Geometry: see drawing. Coordinates: mm, zero at the bounding-box minimum. A direction names the side the tool comes from. Coordinates: 2 decimals unless noted, no trailing zeros. Write each loop counter-clockwise with the first axis right and the second up, starting at its lowest first coordinate (ties: lowest second). Pieces come first, ordered by that corner, then holes. Notation, with made-up numbers: M -30.75,-38 L -4.75,-38 A20 ccw -4.75,-33 Z; hole C -23,-12 d3. An arc over 180 degrees is marked long. Answer as CSV lines item,"result". Start each with the question number.
1. Line query: probe 1 along Y at (x, z) = (22, 16.25) (1 decimal); probe 2 along Y at (x, z) = (8.75, 6.5) (1 decimal); probe 3 along X at (y, z) = (7.5, 13.75) (1 decimal). Output: solid intervals per line, ascending. Write a range as [from, to].
2. Contact query for flat-ended pins moving along their axis: pin 1 Ø1 at (y, z) = (14, 15) entering from +X; pin 2 Ø0.8 at (x, z) = (28, 6.5) entering from +Y (3 decimals); pin 3 Ø1.3 at (y, z) = (12, 10.5) entering from -X; pin 4 Ø1.6 at (x, y) = (2.125, 5.7) entering from +Z. Output: stop coordinate, or through.
3. Section D-D on y = 5.7. Return the cut outline in (x, z) (1 decimal), plus the area to 3 significant figures.
4. Section C-C on x = 24. Return the cut outline in (y, z) (1 decimal).
5. Section A-A on z = 2.25. Count the separate pieces of the cut face and the enclosed holes in it, plus the area to 3 significant figures.
6. Section B-B on y = 14.75. Return the cut outline in (x, z) (1 decimal), plus the area to 3 significant figures.
7. Mould query, pull axis Z, two halves, no side actions, for the marked faces 4, 5 and 6. Classes: pulls with the +Z half, pulls with the -Z half, needs draft (parallel to the pull), parting line crosses it, or undercut.
8. Reachability of the marked faces 1, 2 and 3 from +Z, -Z, +X, -X, +Y, -Y: full face, straight path, thin tool, end or side. Return the list, or none.
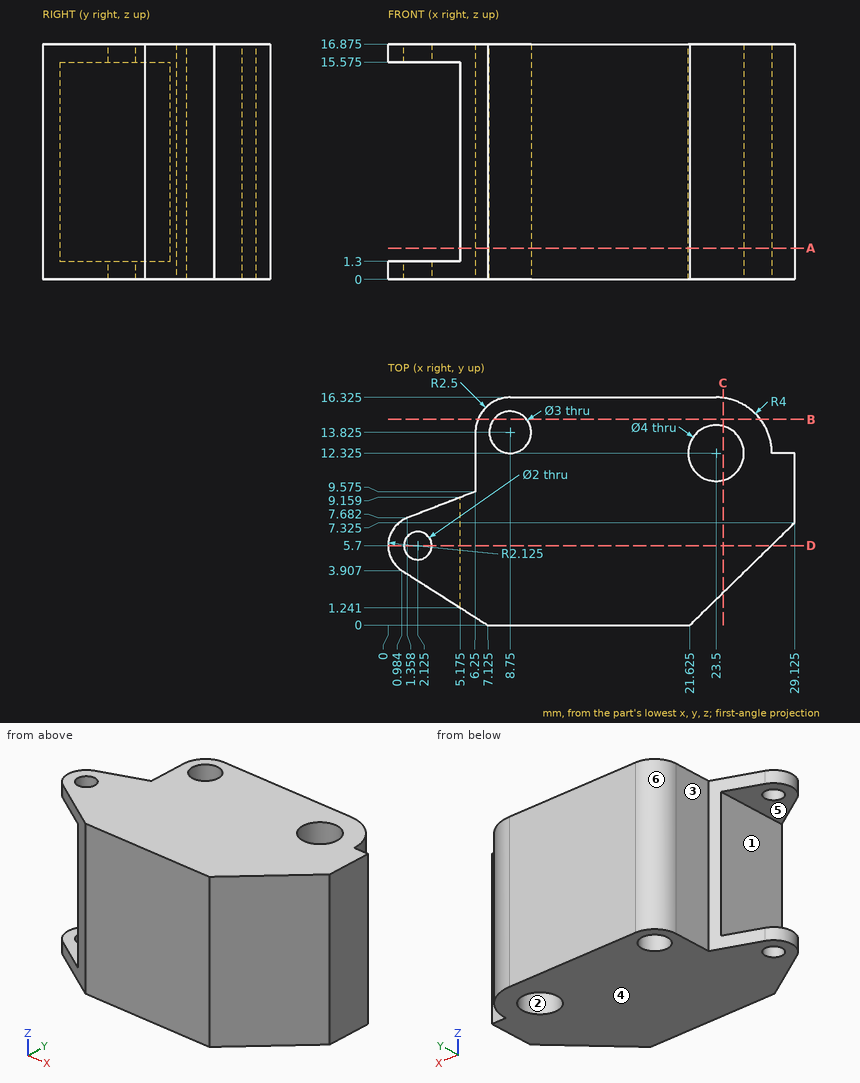
Values:
1,probe 1,"[0.4, 11], [13.6, 16.3]"
1,probe 2,"[0, 12.3], [15.3, 16.3]"
1,probe 3,"[5.2, 29.1]"
2,pin 1,"x = 27.32"
2,pin 2,"y = 12.325"
2,pin 3,"x = 6.25"
2,pin 4,"through"
3,outline,"M 0,0 L 1.1,0 L 1.1,1.3 L 0,1.3 Z; M 0,15.6 L 1.1,15.6 L 1.1,16.9 L 0,16.9 Z; M 3.1,0 L 27.5,0 L 27.5,16.9 L 3.1,16.9 L 3.1,15.6 L 5.2,15.6 L 5.2,1.3 L 3.1,1.3 Z"
3,area,"384 mm²"
4,outline,"M 2.3,0 L 10.4,0 L 10.4,16.9 L 2.3,16.9 Z; M 14.3,0 L 16.3,0 L 16.3,16.9 L 14.3,16.9 Z"
5,separate pieces,"1"
5,enclosed holes,"2"
5,area,"324 mm²"
6,outline,"M 6.4,0 L 7.6,0 L 7.6,16.9 L 6.4,16.9 Z; M 9.9,0 L 26.7,0 L 26.7,16.9 L 9.9,16.9 Z"
6,area,"302 mm²"
7,face 4,"pulls with the -Z half"
7,face 5,"undercut"
7,face 6,"needs draft"
8,face 1,"-X, +Y, -Y"
8,face 2,"+Z, -Z"
8,face 3,"+Z, -Z, -X, +Y"
